Verification items for the finished model (mm, model axes). A direction names the side the tool comes from. Coordinates: 2 decimals unless noted, no trailing zeros. Order: outer loops, then holes, each group sorted by start corner. A loop starts at its lowest first (then second) coordinate and runs counter-clockwise, first axis right, second up.
Q1. Cross-section at D-D, the plane z = 12.7. Record the boundary of the cut face in (x, y) (1 decimal), and give its area (3 significant figures).
Q2. Thickness scan on line 1 (Z direction, x = 0, y = 9.2); line 2 (Y direction, x = -4.5, z = 47.5) (1 decimal). Record the ranges inside material, lowest first.
Q3. Cross-section at C-C, the plane y = 0. Record the boundary of the cut face in (x, z) (1 decimal).
Q4. Cross-section at A-A, the plane y = -6.75. Record the boundary of the cut face in (x, z) (1 decimal).
Q5. Depth check by flat-ended pin: P1, Ø5, axis at y = 0, z = 38.1, coming from the -X side. Enter the tip coordinate at first touch or a pass-through.
Q6. Set-up check for faces 1 (the flat face through (0, 7.938, 38)), 2 (the cylindrical face through (0.1, 8.72, 10.32)), 3 (the cylindrical face through (-8.742, -2.415, 34.951)): record each of +Z, -Z, +X, -X, +Y, -Y from which the full face is reachable in a straight line by a thin tool's end or side.
Q7. Draft check along Y on faces 4 (the cylindrical face through (0.1, -8.74, 61.12)), 5 (the flat face through (7.938, 0, 38)), 6 (the flat face through (-7.938, 5, 38)), 7 (the flat face through (0, -9.525, 38)). Enter one of: pulls with the +Y half, pulls with the -Y half, needs draft (parallel to the pull), parting line crosses it, or undercut.
from build123d import *

# Parameters (mm, degrees)
SKETCH1_W               = 19.05
SKETCH1_H               = 19.05
SKETCH1_W_2             = 15.875
SKETCH1_H_2             = 15.875
BOSS_EXTRUDE1_DEPTH     = 76.2
CUT_EXTRUDE1_DEPTH      = 78.381465804
CUT_EXTRUDE1_DEPTH_BACK = 78.381465804
SKETCH2_R               = 2.38125
CUT_EXTRUDE2_REACH      = 81.121
SKETCH3_R               = 3.96875


with BuildPart() as part:
    # Sketch1 → Boss-Extrude1 (new body)
    with BuildSketch(Plane.XY):
        Rectangle(SKETCH1_W, SKETCH1_H)
        Rectangle(SKETCH1_W_2, SKETCH1_H_2, mode=Mode.SUBTRACT)
    extrude(amount=BOSS_EXTRUDE1_DEPTH)

    # Sketch2 → Cut-Extrude1 (cut, two sides: drawn at the far end of the back side and taken through both)
    with BuildSketch(Plane(origin=(0, 0, 0), x_dir=(1, 0, 0), z_dir=(0, 1, 0)).offset(-CUT_EXTRUDE1_DEPTH_BACK)):
        with Locations(Location((0, -12.7, 0), (0, 0, 270))):
            Circle(SKETCH2_R)
        with Locations(Location((0, -63.5, 0), (0, 0, 270))):
            Circle(SKETCH2_R)
    extrude(amount=CUT_EXTRUDE1_DEPTH + CUT_EXTRUDE1_DEPTH_BACK, mode=Mode.SUBTRACT)

    # Sketch3 → Cut-Extrude2 (cut, up to next)
    with BuildSketch(Plane.ZY.offset(9.525), mode=Mode.PRIVATE) as cut_extrude2_sk1:
        with Locations((38.1, 0)):
            Circle(SKETCH3_R)
    cut_extrude2_tool1 = extrude(cut_extrude2_sk1.sketch, amount=-CUT_EXTRUDE2_REACH, mode=Mode.PRIVATE) & part.part
    add(cut_extrude2_tool1.solids().sort_by_distance((-9.525, 0, 38.1))[0], mode=Mode.SUBTRACT)


solid = part.part
Check values:
1. outline: (-9.5, -9.5) - (-2.4, -9.5) - (-2.4, -7.9) - (-7.9, -7.9) - (-7.9, 7.9) - (-2.4, 7.9) - (-2.4, 9.5) - (-9.5, 9.5) - close; (2.4, -9.5) - (9.5, -9.5) - (9.5, 9.5) - (2.4, 9.5) - (2.4, 7.9) - (7.9, 7.9) - (7.9, -7.9) - (2.4, -7.9) - close
1. area: 95.8 mm2
2. line 1: z = 0 to 10.32, 15.08 to 61.12, 65.88 to 76.2
2. line 2: y = -9.5 to -7.9, 7.9 to 9.5
3. outline: (-9.5, 0) - (-7.9, 0) - (-7.9, 34.1) - (-9.5, 34.1) - close; (-9.5, 42.1) - (-7.9, 42.1) - (-7.9, 76.2) - (-9.5, 76.2) - close; (7.9, 0) - (9.5, 0) - (9.5, 76.2) - (7.9, 76.2) - close
4. outline: (-9.5, 0) - (-7.9, 0) - (-7.9, 76.2) - (-9.5, 76.2) - close; (7.9, 0) - (9.5, 0) - (9.5, 76.2) - (7.9, 76.2) - close
5. P1: stops at x = 7.94
6. face 1: +Z, -Z
6. face 2: +Y, -Y
6. face 3: -X
7. face 4: needs draft
7. face 5: undercut
7. face 6: undercut
7. face 7: pulls with the -Y half
